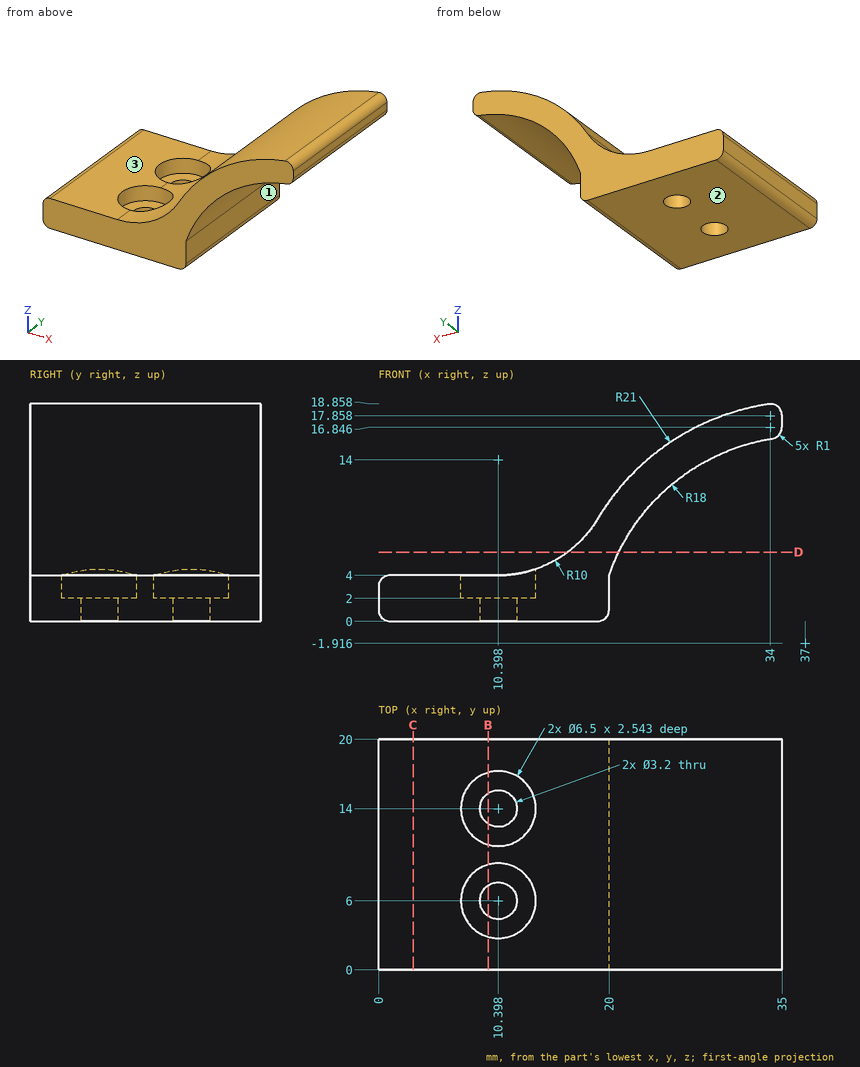
The figure shows three views and two pictorial views of one solid part (mm, origin at its lowest corner). Answer the questions. A direction names the side the tool comes from. Coordinates: 2 decimals unless noted, no trailing zeros. Loops run counter-clockwise (first coordinate to the right, second up) from the corner with the lowest first, then second, coordinate; pieces in that order, holes last. Notation, with made-up numbers: (72.25, 79) - (96.25, 79) arc R17 ccw to (96.25, 98) - close; hole circle Ø1 at (47, 86.25). An arc over 180 degrees is marked (long way). Write item = value, one per line.
1) Section C-C (x = 3) is taken. Determine the outline of the cut face in (y, z).
Responses:
outline = (0, 0) - (20, 0) - (20, 4) - (0, 4) - close
2) Section D-D (z = 6) is taken. Determine the outline of the cut face in (x, y).
Responses:
outline = (16.4, 0) - (20.83, 0) - (20.83, 20) - (16.4, 20) - close
3) Find the intervals of material crossed by line 1 along Y through (x, z) = (8, 3.25) (1 decimal); line 2 along Y through (x, z) = (9, 3) (1 decimal); line 3 along Z through (x, y) = (7, 4), in increasing order.
Responses:
line_1 = 0 to 3.8, 8.2 to 11.8, 16.2 to 20
line_2 = 0 to 3.1, 8.9 to 11.1, 16.9 to 20
line_3 = 0 to 4
4) Each of these flat-tipped pins is pushed along its axis until it touches: P1, Ø1, axis at x = 4.5, y = 14, coming from the +Z side; P2, Ø8, axis at x = 23.5, y = 10, coming from the +Z side; P3, Ø8, axis at x = 20, z = 16.5, coming from the -Y side; P4, Ø10.5, axis at x = 10.4, y = 14, coming from the +Z side. Where does it stop, or does it pass through?
Responses:
P1 = 4
P2 = 16.81
P3 = through
P4 = 5.49
5) Which of the six approach directions +Z, -Z, +X, -X, +Y, -Y give full straight-line access (tool end or side, diameter ignored) to the marked faces 1, 2 and 3?
Responses:
face_1 = -Z, +X, +Y, -Y
face_2 = -Z, +X, -X, +Y, -Y
face_3 = +Z, -X, +Y, -Y
6) Section B-B (x = 9.5) is taken. Determine the outline of the cut face in (y, z) (1 decimal).
Responses:
outline = (0, 0) - (4.7, 0) - (4.7, 2) - (2.9, 2) - (2.9, 4) - (0, 4) - close; (7.3, 0) - (12.7, 0) - (12.7, 2) - (10.9, 2) - (10.9, 4) - (9.1, 4) - (9.1, 2) - (7.3, 2) - close; (15.3, 0) - (20, 0) - (20, 4) - (17.1, 4) - (17.1, 2) - (15.3, 2) - close
